Read the model definition and answer for the solid it produces. Units are mm, in the model's axes. Face numbers are marked on the shaded views. Coordinates: 2 decimals unless noted, no trailing zeros. Loops run counter-clockwise (first coordinate to the right, second up) from the corner with the lowest first, then second, coordinate; pieces in that order, holes last. Notation, with made-up numbers: M 46.5,69.25 L 58.5,69.25 A16 ccw 58.5,100.25 Z; hole C -26.75,33.5 d2. An arc over 180 degrees is marked long. Put each result on its own line as item: value.
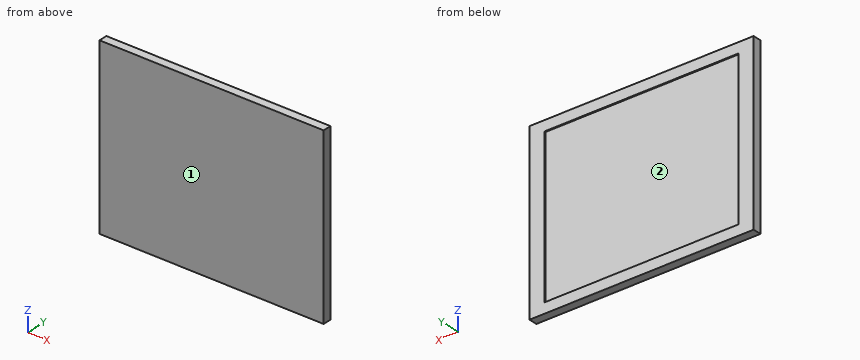
from build123d import *

# Parameters (mm, degrees)
ESBO_O1_W                = 278
ESBO_O1_H                = 216
RESSALTO_EXTRUS_O1_DEPTH = 9.1
ESBO_O2_W                = 240.4
ESBO_O2_H                = 190.7
RESSALTO_EXTRUS_O2_DEPTH = 1.5


with BuildPart() as part:
    # Esboço1 → Ressalto-extrusão1 (new body)
    with BuildSketch(Plane(origin=(0, 0, 0), x_dir=(1, 0, 0), z_dir=(0, 1, 0))):
        Rectangle(ESBO_O1_W, ESBO_O1_H)
    extrude(amount=RESSALTO_EXTRUS_O1_DEPTH)

    # Esboço2 → Ressalto-extrusão2 (add)
    with BuildSketch(Plane(origin=(0, 9.1, 0), x_dir=(1, 0, 0), z_dir=(0, 1, 0))):
        Polygon((-139, 108), (-120.2, 108), (120.2, 108), (139, 108), (139, -108), (120.2, -108), (-120.2, -108), (-139, -108), align=None)
        Rectangle(ESBO_O2_W, ESBO_O2_H, mode=Mode.SUBTRACT)
    extrude(amount=RESSALTO_EXTRUS_O2_DEPTH)


solid = part.part
1) Straight lines are drawn through the part: line 1 (X direction, y = 10.25, z = 12); line 2 (Z direction, x = 106, y = 9.5); line 3 (Y direction, x = 29, z = 49.5). For each, find the intervals that lie inside material, in ascending order. Write a range as [from, to].
Answer list:
line 1: x = [-139, -120.2], [120.2, 139]
line 2: z = [-108, -95.35], [95.35, 108]
line 3: y = [0, 9.1]
2) Given pin 1 Ø3 at (x, z) = (2.5, -24.5) entering from -Y; pin 2 Ø8 at (x, z) = (-110.5, 21.5) entering from +Y, each flat-ended and moving along its own axis, determine where each tip first touches the part or whether it passes through.
Answer list:
pin 1: stops at y = 0
pin 2: stops at y = 9.1
3) Determine the mould class of the marked faces 1 and 2 for opening direction X: released by +X, released by -X, zero draft, split by the parting line, or undercut.
Answer list:
face 1: zero draft
face 2: undercut
4) Find section B-B, the plane z = 0. Write down the section's boundary in (x, y).
Answer list:
outline: M -139,0 L 139,0 L 139,10.6 L 120.2,10.6 L 120.2,9.1 L -120.2,9.1 L -120.2,10.6 L -139,10.6 Z
5) Find section A-A, the plane x = 57.5. Write down the section's boundary in (y, z), plus the area to 3 significant figures.
Answer list:
outline: M 0,-108 L 10.6,-108 L 10.6,-95.35 L 9.1,-95.35 L 9.1,95.35 L 10.6,95.35 L 10.6,108 L 0,108 Z
area: 2,000 mm^2
